The listing builds one solid part. Answer for the finished solid, in the listing's coordinates (mm). A direction names the side the tool comes from. Coordinates: 2 decimals unless noted, no trailing zeros. Write each loop counter-clockwise with the first axis right and the second up, starting at its lowest first coordinate (ties: lowest second). Pieces come first, ordered by that corner, then holes.
Autodesk Inventor part; units mm, degrees
ref_plane "XZ Plane" through (0, 0, 0) normal (0, 1, 0) x (-1, 0, 0)
ref_plane "XY Plane" through (0, 0, 0) normal (0, 0, 1) x (1, 0, 0)
sketch "Sketch1" plane through (0, 0, 0) normal (0, 0, 1) x (1, 0, 0)
  line L0 (0, 0) -> (203.2, 0)
  line L1 (203.2, 0) -> (203.2, 50.8)
  line L2 (152.4, 101.6) -> (50.8, 101.6)
  line L3 (0, 50.8) -> (0, 0)
  line L4 (50.8, 101.6) -> (0, 50.8)
  line L5 (152.4, 101.6) -> (203.2, 50.8)
  point P0 (203.2, 101.6)
  point P1 (0, 101.6)
  dimension "d0" = 50.8
  dimension "d1" = 50.8
  dimension "d2" = 50.8
  dimension "d3" = 50.8
  dimension "d7" = 203.2
  dimension "d8" = 101.6
extrude "Extrusion1" add sketch "Sketch1" along normal blind 6.35
sketch "Sketch2" plane through (0, 0, 6.35) normal (0, 0, 1) x (1, 0, 0)
  line L0 (0, 0) -> (203.2, 0)
  line L1 (0, 0) -> (203.2, 0)
  line L2 (203.2, 0) -> (203.2, 50.8)
  line L3 (203.2, 50.8) -> (152.4, 101.6)
  line L4 (152.4, 101.6) -> (50.8, 101.6)
  line L5 (50.8, 101.6) -> (0, 50.8)
  line L6 (0, 50.8) -> (0, 0)
  point P0 (25.4, 12.7)
  point P1 (76.1155, 12.7)
  dimension "d6" = 12.7
  dimension "d9" = 25.4
hole "Hole1" at (25.4, 12.7, 6.35) at (76.1155, 12.7, 6.35) direction (0, 0, -1) diameter 12.7 depth 25.4 tip angle 118
pattern_linear "Rectangular Pattern1" count 4 spacing 50.8 along (1, 0, 0) of "Hole1" first direction both ways yes
sketch "Sketch3" plane through (0, 0, 6.35) normal (0, 0, 1) x (1, 0, 0)
  line L0 (0, 0) -> (203.2, 0)
  line L1 (203.2, 0) -> (203.2, 50.8)
  line L2 (203.2, 50.8) -> (152.4, 101.6)
  line L3 (152.4, 101.6) -> (50.8, 101.6)
  line L4 (50.8, 101.6) -> (0, 50.8)
  line L5 (0, 50.8) -> (0, 0)
  arc A0 (76.1577, 6.3501) -> (76.1577, 19.0499) centre (76.2, 12.7) ccw
  arc A1 (76.1577, 19.0499) -> (76.1577, 6.3501) centre (76.1155, 12.7) ccw
  circle A2 centre (177.7155, 12.7) radius 6.35
  arc A3 (126.9577, 6.3501) -> (126.9577, 19.0499) centre (127, 12.7) ccw
  arc A4 (126.9577, 19.0499) -> (126.9577, 6.3501) centre (126.9155, 12.7) ccw
  arc A5 (25.3577, 19.0499) -> (25.3577, 6.3501) centre (25.3155, 12.7) ccw
  arc A6 (25.3577, 6.3501) -> (25.3577, 19.0499) centre (25.4, 12.7) ccw
  line L6 (140.7734, 84.608) -> (140.7734, 58.6856) construction
  line L7 (152.4, 101.6) -> (50.8, 101.6)
  line L8 (137.5984, 84.608) -> (137.5984, 58.6856)
  line L9 (143.9484, 58.6856) -> (143.9484, 84.608)
  arc A7 (143.9484, 84.608) -> (137.5984, 84.608) centre (140.7734, 84.608) ccw
  arc A8 (137.5984, 58.6856) -> (143.9484, 58.6856) centre (140.7734, 58.6856) ccw
  point P0 (140.7734, 71.6468)
  point P1 (174.2566, 38.1636)
  point P2 (149.4142, 41.0439)
  dimension "d20" = 6.35
hole "Hole2" at (174.2566, 38.1636, 6.35) at (149.4142, 41.0439, 6.35) direction (0, 0, -1) diameter 4.9784 depth 19.05 tip angle 118
extrude "Extrusion2" cut sketch "Sketch3" against normal blind 6.35 contours A7 L9 A8 L8
sketch "Sketch4" plane through (0, 0, 0) normal (0, 0, -1) x (-1, 0, 0)
  arc A0 (-143.9484, 58.6856) -> (-137.5984, 58.6856) centre (-140.7734, 58.6856) ccw
  line L0 (-143.9484, 58.6856) -> (-143.9484, 84.608)
  arc A1 (-137.5984, 84.608) -> (-143.9484, 84.608) centre (-140.7734, 84.608) ccw
  line L1 (-137.5984, 84.608) -> (-137.5984, 58.6856)
  circle A2 centre (-174.2566, 38.1636) radius 2.4892
  circle A3 centre (-149.4142, 41.0439) radius 2.4892
  line L2 (0, 0) -> (-203.2, 0)
  line L3 (0, 50.8) -> (0, 0)
  line L4 (-50.8, 101.6) -> (0, 50.8)
  line L5 (-152.4, 101.6) -> (-50.8, 101.6)
  line L6 (-203.2, 50.8) -> (-152.4, 101.6)
  line L7 (-203.2, 0) -> (-203.2, 50.8)
  arc A4 (-25.3577, 6.3501) -> (-25.3577, 19.0499) centre (-25.3155, 12.7) ccw
  arc A5 (-25.3577, 19.0499) -> (-25.3577, 6.3501) centre (-25.4, 12.7) ccw
  circle A6 centre (-177.7155, 12.7) radius 6.35
  arc A7 (-126.9577, 19.0499) -> (-126.9577, 6.3501) centre (-127, 12.7) ccw
  arc A8 (-126.9577, 6.3501) -> (-126.9577, 19.0499) centre (-126.9155, 12.7) ccw
  arc A9 (-76.1577, 19.0499) -> (-76.1577, 6.3501) centre (-76.2, 12.7) ccw
  arc A10 (-76.1577, 6.3501) -> (-76.1577, 19.0499) centre (-76.1155, 12.7) ccw
  line L8 (-152.4, 101.6) -> (-50.8, 101.6)
  line L9 (-101.6, 101.6) -> (-101.6, 0)
  line L10 (0, 0) -> (-203.2, 0)
ref_plane "Work Plane1" through (101.6, 101.6, 0) normal (1, 0, 0) x (0, -1, 0)
mirror "Mirror1" about plane through (101.6, 101.6, 0) normal (1, 0, 0) of "Extrusion2", "Hole2"
mirror "Mirror2" about plane through (101.6, 101.6, 0) normal (1, 0, 0) of "Extrusion1", "Extrusion2", "Hole2", "Mirror1", "Hole1", "Rectangular Pattern1"
sketch "Sketch5" plane through (0, 0, 0) normal (0, 0, -1) x (-1, 0, 0)
  line L0 (-91.0569, 50.3137) -> (-46.6879, 50.3137) construction
  line L1 (-46.6879, 50.3137) -> (-46.6879, 47.0459) construction
  line L2 (-46.6879, 47.0459) -> (-91.0569, 47.0459) construction
  line L3 (-91.0569, 47.0459) -> (-91.0569, 50.3137) construction
  point P0 (0, 0)
properties part number "junk" material "Water"
1. Section D-D on x = 72.5 is taken. Give the vertices of the cut face in (y, z).
Results found:
outline: (0, 0) - (7.54, 0) - (7.54, 6.35) - (0, 6.35) - close; (17.86, 0) - (101.6, 0) - (101.6, 6.35) - (17.86, 6.35) - close
2. A tool of negligible diameter and unlimited length cuts with its end or side. For faces 1 (the cylindrical face through (140.843, 87.782, 3.219)), 2 (the flat face through (102, 101.6, 3)), from which of +Z, -Z, +X, -X, +Y, -Y can it reach the whole face along a straight path? Write none if from no direction.
Results found:
face 1: +Z, -Z
face 2: +Z, -Z, +X, -X, +Y
3. For a pull along Y with two mould halves and no side action, classify faces 3 (the flat face through (100, 52, 6.35)), 4 (the flat face through (143.948, 71, 3)), 5 (the flat face through (25.8, 76.6, 3.1)) as pulls with the +Y half, pulls with the -Y half, needs draft (parallel to the pull), parting line crosses it, or undercut.
Results found:
face 3: needs draft
face 4: undercut
face 5: pulls with the +Y half
4. Find the intervals of material crossed by L1, parallel to X at y = 12.7, z = 4.75; L2, parallel to Y at x = 176, z = 1.5; L3, parallel to X at y = 85.5, z = 5.5, in increasing order.
Results found:
L1: x = 0 to 19.13, 31.83 to 69.85, 82.63 to 120.65, 133.43 to 171.45, 184.23 to 203.2
L2: y = 0 to 6.61, 18.79 to 36.39, 39.94 to 78
L3: x = 34.7 to 59.38, 65.47 to 137.73, 143.82 to 168.5
5. Section B-B on y = 12.7 is taken. Give the vertices of the cut face in (x, z), then the cut area to 3 significant figures.
Results found:
outline: (0, 0) - (19.13, 0) - (19.13, 6.35) - (0, 6.35) - close; (31.83, 0) - (69.85, 0) - (69.85, 6.35) - (31.83, 6.35) - close; (82.63, 0) - (120.65, 0) - (120.65, 6.35) - (82.63, 6.35) - close; (133.43, 0) - (171.45, 0) - (171.45, 6.35) - (133.43, 6.35) - close; (184.23, 0) - (203.2, 0) - (203.2, 6.35) - (184.23, 6.35) - close
area: 966 mm2
6. Flat-ended cylindrical pins translate along their axes: P1, Ø1.5, axis at x = 164, z = 2, coming from the -Y side; P2, Ø1.9, axis at y = 73, z = 4, coming from the +X side; P3, Ø1.9, axis at y = 71, z = 3.5, coming from the -X side; P4, Ø1.5, axis at y = 82, z = 2, coming from the +X side. Find the tip coordinate at first contact, or state that the pin passes through.
Results found:
P1: stops at y = 0
P2: stops at x = 181.95
P3: stops at x = 19.25
P4: stops at x = 172.75
7. Section A-A on y = 61 is taken. Give the vertices of the cut face in (x, z), then the cut area to 3 significant figures.
Results found:
outline: (10.2, 0) - (59.25, 0) - (59.25, 6.35) - (10.2, 6.35) - close; (65.6, 0) - (137.6, 0) - (137.6, 6.35) - (65.6, 6.35) - close; (143.95, 0) - (193, 0) - (193, 6.35) - (143.95, 6.35) - close
area: 1,080 mm2
8. Section C-C on z = 2.75 is taken. State how many separate pieces and enclosed holes the cut face has, then the cut area to 3 significant figures.
Results found:
separate pieces: 1
enclosed holes: 10
area: 17,100 mm2
